The drawing under review shows one solid part. Ordinate dimensions are in mm from its lowest x, y, z. A direction names the side the tool comes from. Coordinates: 2 decimals unless noted, no trailing zeros. Loops run counter-clockwise (first coordinate to the right, second up) from the corner with the lowest first, then second, coordinate; pieces in that order, holes last. Notation, with made-up numbers: M -35.75,57.25 L -26.75,57.25 A11 ccw -26.75,75.25 Z; hole C 8.25,10 d1. An arc over 180 degrees is marked long. Return JSON: item names as keys, results as strings.
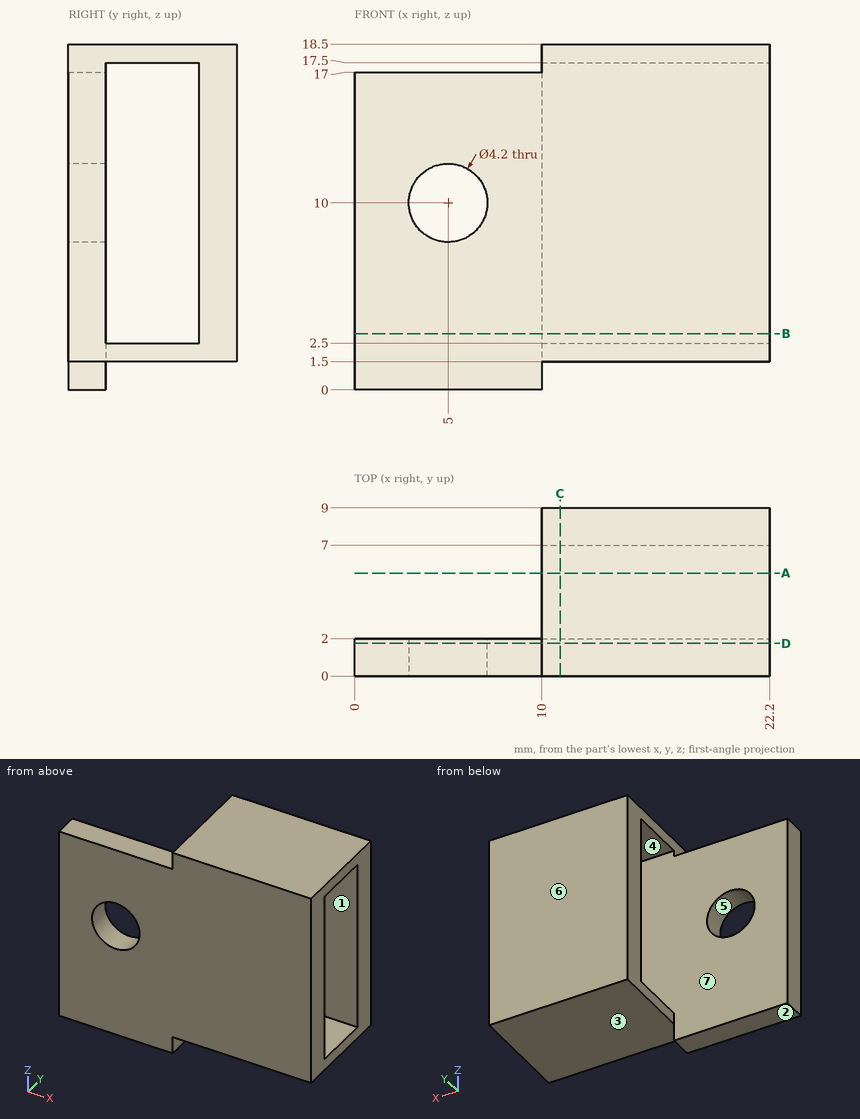
1. The part is to be moulded in two halves that separate along Y. For the marked faces 4, 5, 6 and 7, say which applies: released by +Y, released by -Y, zero draft, split by the parting line, or undercut.
Check values:
{"face 4": "undercut", "face 5": "zero draft", "face 6": "released by +Y", "face 7": "undercut"}
2. Add section D-D on y = 1.75. Give the boundary of the cut face in (x, z), plus the area to 3 significant figures.
Check values:
{"outline": "M 0,0 L 10,0 L 10,1.5 L 22.2,1.5 L 22.2,18.5 L 10,18.5 L 10,17 L 0,17 Z; hole C 5,10 d4.2", "area": "364 mm²"}
3. Add section A-A on y = 5.5. Give the boundary of the cut face in (x, z).
Check values:
{"outline": "M 10,1.5 L 22.2,1.5 L 22.2,2.5 L 10,2.5 Z; M 10,17.5 L 22.2,17.5 L 22.2,18.5 L 10,18.5 Z"}
4. To check wall thickness, follow line 1 (Y direction, x = 17.75, z = 15.75); line 2 (Z direction, x = 5, y = 0.6); line 3 (X direction, y = 0.8, z = 10). State the ranges of each line that lie inside material, in increasing order.
Check values:
{"line 1": "0 to 2, 7 to 9", "line 2": "0 to 7.9, 12.1 to 17", "line 3": "0 to 2.9, 7.1 to 22.2"}
5. Machinability: for the marked faces 1, 2 and 3, which of the approach directions +Z, -Z, +X, -X, +Y, -Y give a long, thin tool a straight path to every point of the face, cutting with its end or side? Answer none if there is none.
Check values:
{"face 1": "+X, -X", "face 2": "-Z, +X, -X, +Y, -Y", "face 3": "-Z, +X, +Y, -Y"}
6. Insertion check: pin 1 Ø1 at (x, y) = (6.5, 1) entering from +Z; pin 2 Ø4.5 at (y, z) = (6, 14) entering from -X; pin 3 Ø5.5 at (x, z) = (5, 10) entering from +Y. Each pin has a flat end and moves straight along its axis. Give the tip position at first contact, or say it passes through.
Check values:
{"pin 1": "z = 17", "pin 2": "x = 10", "pin 3": "y = 2"}
7. Add section B-B on z = 3. Give the boundary of the cut face in (x, y).
Check values:
{"outline": "M 0,0 L 22.2,0 L 22.2,2 L 0,2 Z; M 10,7 L 22.2,7 L 22.2,9 L 10,9 Z"}
8. Add section C-C on x = 11. Give the boundary of the cut face in (y, z).
Check values:
{"outline": "M 0,1.5 L 9,1.5 L 9,18.5 L 0,18.5 Z; hole M 2,2.5 L 7,2.5 L 7,17.5 L 2,17.5 Z"}
